Print and shaded views of the part. All mm, measured from the part's lowest x, y and z. A direction names the side the tool comes from. Round coordinates to 2 decimals unless told otherwise and drop trailing zeros. Loops run counter-clockwise (first coordinate to the right, second up) from the corner with the lowest first, then second, coordinate; pieces in that order, holes last. Notation, with made-up numbers: (44.5, -10) - (48.5, -10) arc R32 cw to (48.5, 22) - close; hole circle Ø1 at (-30, 80). An arc over 180 degrees is marked (long way). Answer as a JSON object with one key per item and string values.
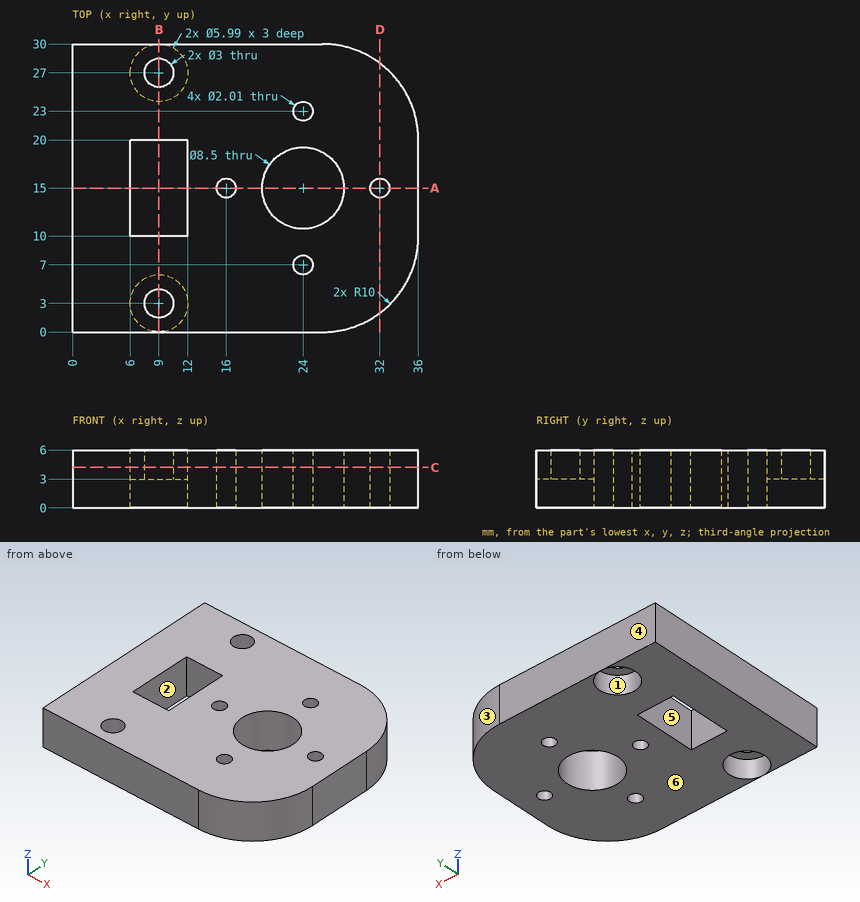
1) Slice it at D-D on x = 32. List the corners of the cut face in (y, z) (3 decimals), then the cut area to 3 significant figures.
Values follow:
{"outline": "(2, 0) - (13.995, 0) - (13.995, 6) - (2, 6) - close; (16.005, 0) - (28, 0) - (28, 6) - (16.005, 6) - close", "area": "144 mm²"}
2) Probe probe 1 along Y at (x, z) = (9, 4.45); probe 2 along Y at (x, z) = (24, 1.8) (3 decimals); probe 3 along Y at (x, z) = (16, 1.05) (3 decimals). List the from-to ranges inside material, lowest first.
Values follow:
{"probe 1": "0 to 1.5, 4.5 to 10, 20 to 25.5, 28.5 to 30", "probe 2": "0 to 5.995, 8.005 to 10.75, 19.25 to 21.995, 24.005 to 30", "probe 3": "0 to 13.995, 16.005 to 30"}
3) Slice it at C-C on z = 4.2. Count the separate pieces of the cut face and the enclosed holes in it, then the cut area to 3 significant figures.
Values follow:
{"separate pieces": "1", "enclosed holes": "8", "area": "894 mm²"}
4) Two-plate mould, pull along Y, no slides. Class the marked faces 4, 5 and 6: pulls with the +Y half, pulls with the -Y half, needs draft (parallel to the pull), parting line crosses it, or undercut.
Values follow:
{"face 4": "pulls with the +Y half", "face 5": "undercut", "face 6": "needs draft"}
5) Slice it at B-B on x = 9. List the corners of the cut face in (y, z) (3 decimals).
Values follow:
{"outline": "(0, 0) - (0.005, 0) - (0.005, 3) - (1.5, 3) - (1.5, 6) - (0, 6) - close; (4.5, 3) - (5.995, 3) - (5.995, 0) - (10, 0) - (10, 6) - (4.5, 6) - close; (20, 0) - (24.005, 0) - (24.005, 3) - (25.5, 3) - (25.5, 6) - (20, 6) - close; (28.5, 3) - (29.995, 3) - (29.995, 0) - (30, 0) - (30, 6) - (28.5, 6) - close"}
6) Tool access for the marked faces 1, 2 and 3: list every direction of +Z, -Z, +X, -X, +Y, -Y with a clear straight run to the whole face (end or side of a thin tool).
Values follow:
{"face 1": "-Z", "face 2": "+Z, -Z", "face 3": "+Z, -Z, +X, +Y"}
7) Slice it at A-A on y = 15. List the corners of the cut face in (x, z) (3 decimals), then the cut area to 3 significant figures.
Values follow:
{"outline": "(0, 0) - (6, 0) - (6, 6) - (0, 6) - close; (12, 0) - (14.995, 0) - (14.995, 6) - (12, 6) - close; (17.005, 0) - (19.75, 0) - (19.75, 6) - (17.005, 6) - close; (28.25, 0) - (30.995, 0) - (30.995, 6) - (28.25, 6) - close; (33.005, 0) - (36, 0) - (36, 6) - (33.005, 6) - close", "area": "105 mm²"}
